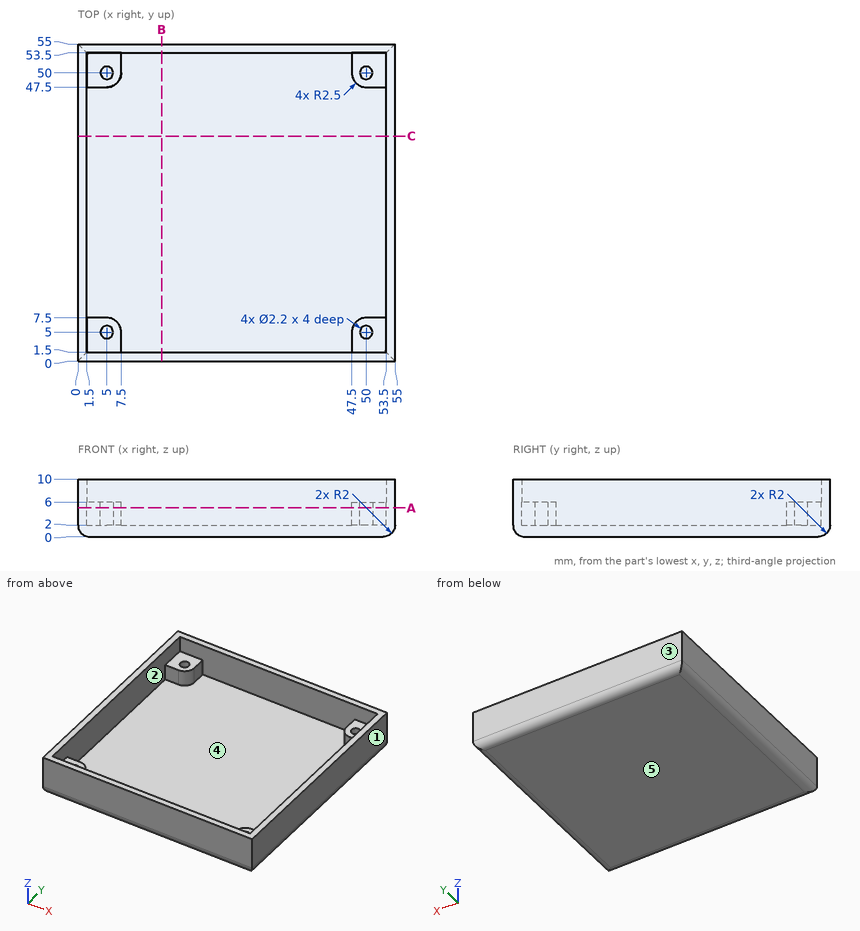
Source: three-view drawing plus pictorial views. Frame: mm from the lowest corner of the part. A direction names the side the tool comes from. Coordinates: 2 decimals unless noted, no trailing zeros. Order: outer loops, then holes, each group sorted by start corner. A loop starts at its lowest first (then second) coordinate and runs counter-clockwise, first axis right, second up. Notation, with made-up numbers: M 83,31.5 L 103,31.5 A24 cw 103,47.5 Z; hole C 46,24.25 d1. An arc over 180 degrees is marked long. Write each question's results on one line, items separated by ' | '. Start each with the question number.
1. Draft query along Y for the marked faces 1, 2 and 3. Return one class per face: +Y half, -Y half, draft (parallel to the pull), parting line (faces both ways), or undercut.
2. Pin query (flat end, axial travel): pin 1 (1.1 mm diameter, centred on x = 5, y = 5.5, fed in from +Z); pin 2 (1.8 mm diameter, centred on x = 5, y = 3, fed in from +Z). Return the tip coordinate at first contact, or that it passes through.
3. Reachability of the marked faces 4 and 5 from +Z, -Z, +X, -X, +Y, -Y: full face, straight path, thin tool, end or side. Return the list, or none.
4. Section B-B, the plane x = 14.5. Return the cut outline in (y, z).
5. Section A-A, the plane z = 5. Return the cut outline in (x, y).
6. Material intervals for L1, parallel to Y at x = 5, z = 5.15; L2, parallel to Y at x = 18, z = 3.75, sorted ascending.
Solution:
1) face 1: draft | face 2: undercut | face 3: +Y half
2) pin 1: z = 2 | pin 2: z = 6
3) face 4: +Z | face 5: -Z, +X, -X, +Y, -Y
4) outline: M 0,2 A2 ccw 2,0 L 53,0 A2 ccw 55,2 L 55,10 L 53.5,10 L 53.5,2 L 1.5,2 L 1.5,10 L 0,10 Z
5) outline: M 0,0 L 55,0 L 55,55 L 0,55 Z; hole M 1.5,7.5 L 5,7.5 A2.5 cw 7.5,5 L 7.5,1.5 L 47.5,1.5 L 47.5,5 A2.5 cw 50,7.5 L 53.5,7.5 L 53.5,47.5 L 50,47.5 A2.5 cw 47.5,50 L 47.5,53.5 L 7.5,53.5 L 7.5,50 A2.5 cw 5,47.5 L 1.5,47.5 Z; hole C 5,5 d2.2; hole C 5,50 d2.2; hole C 50,5 d2.2; hole C 50,50 d2.2
6) L1: 0 to 3.9, 6.1 to 7.5, 47.5 to 48.9, 51.1 to 55 | L2: 0 to 1.5, 53.5 to 55
